Part model, mm, in its own coordinate system. A direction names the side the tool comes from. Round coordinates to 2 decimals unless told otherwise and drop trailing zeros. Write each loop counter-clockwise with the first axis right and the second up, starting at its lowest first coordinate (ties: lowest second). Pieces come first, ordered by that corner, then holes.
from build123d import *

# Parameters (mm, degrees)
SKETCH_5_R             = 7.5
SKETCH_5_R_2           = 5.25
EXTRUDE_1_DEPTH        = 3.5
SKETCH_6_R             = 1.25
CUT_EXTRUDE_M3_1_DEPTH = 42.856899073
CHAMFER_1_SIZE         = 0.5
CHAMFER_2_SIZE         = 1
CUT_EXTRUDE_14_DEPTH   = 3.5
FILLET_2_R             = 2.25
HOLE_WIZARD_M3_1_D     = 2.5


with BuildPart() as part:
    # 草图1 → 旋转1 (revolve)
    with BuildSketch(Plane(origin=(0, 0, 0), x_dir=(0, 0, -1), z_dir=(1, 0, 0))):
        Polygon((-7.5, 0), (-5.25, 0), (-5.25, 18), (0, 18), (0, 28), (-22, 28), (-22, 21), (-9, 21), (-9, 18), (-7.5, 18), align=None)
    revolve(axis=Axis((0, 28, 0), (0, -1, 0)))

    # 草图5 → 凸台-拉伸1 (add)
    with BuildSketch(Plane.XZ):
        with Locations(Location((0, 0, 0), (0, 0, 90))):
            Circle(SKETCH_5_R)
        with Locations(Location((0, 0, 0), (0, 0, 90))):
            Circle(SKETCH_5_R_2, mode=Mode.SUBTRACT)
    extrude(amount=EXTRUDE_1_DEPTH)

    # 草图6 → M3螺纹孔1 (cut, through all)
    with BuildSketch(Plane.XY):
        with Locations(Location((0, 7.5, 0), (0, 0, 270))):
            Circle(SKETCH_6_R)
    extrude(amount=CUT_EXTRUDE_M3_1_DEPTH, mode=Mode.SUBTRACT)

    # 倒角1
    chamfer_1_edges = [part.edges().sort_by_distance(p)[0] for p in [
        (0, -3.5, -7.5),
        (0, 18, -9),
    ]]
    chamfer(chamfer_1_edges, length=CHAMFER_1_SIZE)

    # 倒角2
    chamfer_2_edges = [part.edges().sort_by_distance(p)[0] for p in [
        (0, 28, -22),
        (0, 21, -22),
    ]]
    chamfer(chamfer_2_edges, length=CHAMFER_2_SIZE)

    # 草图8 → 切除-拉伸14 (cut)
    with BuildSketch(Plane.XZ.offset(-21)):
        with BuildLine():
            Line((-9.866772518, 3.591211505), (-14.095389312, 5.13030215))
            ThreePointArc((-14.095389312, 5.13030215), (0, -15), (14.095389312, 5.13030215))
            Line((14.095389312, 5.13030215), (9.866772518, 3.591211505))
            ThreePointArc((9.866772518, 3.591211505), (0, -10.5), (-9.866772518, 3.591211505))
        make_face()
    extrude(amount=-CUT_EXTRUDE_14_DEPTH, mode=Mode.SUBTRACT)

    # 圆角2
    fillet_2_edges = [part.edges().sort_by_distance(p)[0] for p in [
        (9.866772518, 22.75, 3.591211505),
        (14.095389312, 22.75, 5.13030215),
        (-9.866772518, 22.75, 3.591211505),
        (-14.095389312, 22.75, 5.13030215),
    ]]
    fillet(fillet_2_edges, radius=FILLET_2_R - 0.0001)  # a hair under: the kernel refuses the full size

    # M3 螺纹孔1 (through all)
    with Locations(Plane(origin=(0, 28, -18), x_dir=(0, 0, 1), z_dir=(0, 1, 0))):
        with Locations((0, 0), (18, 18), (36, 0), (18, -18)):
            Hole(HOLE_WIZARD_M3_1_D / 2)


solid = part.part
Q1. Saw through at B-B, the plane z = 0. Give the number of separate pieces and of enclosed holes in the cut face, and give its area (3 significant figures).
Q2. Wall check: line 1 (X direction, y = 23.3, z = 0); line 2 (Z direction, x = -1, y = 27); line 3 (Y direction, x = 7, z = -15). Give the ranges that are in metal, low to high.
Q3. Two-plate mould, pull along X, no slides. Class faces 1 (the cylindrical face through (-0.479, 24.451, 16.845)), 2 (the flat face through (4, 21, 9)), 3 (the cylindrical face through (10.627, 22.774, 3.325)), 4 (the cylindrical face through (21.477, 24.465, -4.769)): released by +X, released by -X, zero draft, split by the parting line, or undercut.
Q4. Saw through at A-A, the plane y = 17. Write the cut outline in (x, z), and give its area (3 significant figures).
Q5. Tool access for faces 5 (the cylindrical face through (-16.946, 24.451, -0.672)), 6 (the cylindrical face through (-8.923, 19.732, -1.172)): list every direction of +Z, -Z, +X, -X, +Y, -Y with a clear straight run to the whole face (end or side of a thin tool).
Q6. Saw through at C-C, the plane y = 7.5. Write the cut outline in (x, z).
Q7. Drop flat-ended pins along their axis: P1, Ø3, axis at x = 0, y = 7.5, coming from the -Z side; P2, Ø10, axis at x = -5, y = 17, coming from the -Z side; P3, Ø3, axis at x = -14.5, y = 24.5, coming from the -Z side. Give the stop position or say it passes through.
Computed:
1. separate pieces: 3
1. enclosed holes: 0
1. area: 390 mm2
2. line 1: x = -22 to -19.25, -16.75 to -15, -10.5 to 10.5, 15 to 16.75, 19.25 to 22
2. line 2: z = -21.98 to -18.75, -17.25 to 17.25, 18.75 to 21.98
2. line 3: y = 21 to 28
3. face 1: undercut
3. face 2: zero draft
3. face 3: undercut
3. face 4: split by the parting line
4. outline: circle Ø15 at (0, 0); hole circle Ø10.5 at (0, 0)
4. area: 90.1 mm2
5. face 5: +Y, -Y
5. face 6: -Y
6. outline: (-1.25, 5.1) - (-1.25, 7.4) arc R7.5 ccw (long way) to (1.25, 7.4) - (1.25, 5.1) arc R5.25 cw (long way) to start
7. P1: stops at z = -7.5
7. P2: stops at z = -21.53
7. P3: stops at z = -17.75
